Autodesk Inventor part; units mm, degrees
ref_plane "YZ Plane" through (0, 0, 0) normal (1, 0, 0) x (0, 1, 0)
ref_plane "XZ Plane" through (0, 0, 0) normal (0, 1, 0) x (-1, 0, 0)
ref_plane "XY Plane" through (0, 0, 0) normal (0, 0, 1) x (1, 0, 0)
sketch "Sketch1" plane through (0, 0, 0) normal (0, 0, 1) x (1, 0, 0)
  line L0 (0, 0) -> (-1.5, 0)
  line L1 (-1.5, 0) -> (-1.5, 7)
  line L2 (-1.5, 7) -> (-1.5, 7)
  line L3 (-1.5, 7) -> (-1.5, 8)
  line L4 (-1.5, 8) -> (-3, 8)
  line L5 (-3, 8) -> (-3, 10)
  line L6 (-3, 10) -> (0, 10)
  line L7 (0, 10) -> (0, 0)
  dimension "d0" = 2
  dimension "d1" = 3
  dimension "d2" = 1.5
  dimension "d3" = 0
  dimension "d4" = 1
  dimension "d5" = 10
  dimension "d6" = 90
revolve "Revolution1" add sketch "Sketch1" angle 360 about axis through (0, 10, 0) along (0, -1, 0)
thread "Thread1"
sketch "Sketch2" plane through (0, 10, 0) normal (0, 1, 0) x (1, 0, 0)
  line L0 (5, 0.35) -> (-5, 0.35)
  line L1 (-5, 0.35) -> (-5, -0.35)
  line L2 (-5, -0.35) -> (5, -0.35)
  line L3 (5, -0.35) -> (5, 0.35)
  line L4 (5, 0.35) -> (-5, -0.35) construction
  line L5 (-5, 0.35) -> (5, -0.35) construction
  point P0 (0, 0)
  dimension "d10" = 10
  dimension "d11" = 0.7
fillet "Fillet1" radius 0.25 1 edges at (3, 10, 0)
extrude "Extrusion2" cut sketch "Sketch2" against normal blind 0.7
fillet "Fillet2" radius 0.3 1 edges at (1.5, 8, 0)
properties part number "TorsionOscillator-Screw-M3-Brass-CheeseHead-8mm-Std" material "Brass, Soft Yellow"
Part model, mm, in its own coordinate system. A direction names the side the tool comes from. Give positions to 0.01 mm unless a question says otherwise; leave off trailing zeros. Order: outer loops, then holes, each group sorted by start corner. A loop starts at its lowest first (then second) coordinate and runs counter-clockwise, first axis right, second up. Notation, with made-up numbers: (20, 68) - (78, 68) arc R26 cw to (78, 85) - close; hole circle Ø6 at (63.5, -19.75). An arc over 180 degrees is marked (long way). One line per question, with ' | ' between items.
1. Band-saw the part on A-A on x = 0. List the corners of the cut face in (y, z).
Filled in:
outline: (0, -1.5) - (7.7, -1.5) arc R0.3 cw to (8, -1.8) - (8, -3) - (9.75, -3) arc R0.25 ccw to (10, -2.75) - (10, -0.35) - (9.3, -0.35) - (9.3, 0.35) - (10, 0.35) - (10, 2.75) arc R0.25 ccw to (9.75, 3) - (8, 3) - (8, 1.8) arc R0.3 cw to (7.7, 1.5) - (0, 1.5) - close
2. Drill centre lines: probe 1 along Y at (x, z) = (-1.05, 1.75); probe 2 along Y at (x, z) = (-0.9, 0); probe 3 along X at (y, z) = (7.5, 0.75). Where is each one in solid material? Low to high.
Filled in:
probe 1: 8 to 10 | probe 2: 0 to 9.3 | probe 3: -1.3 to 1.3
3. Band-saw the part on C-C on y = 1. List the corners of the cut face in (x, z), then the cut area to 3 significant figures.
Filled in:
outline: circle Ø3 at (0, 0) | area: 7.07 mm²
4. Band-saw the part on B-B on z = 0. List the corners of the cut face in (x, y).
Filled in:
outline: (-3, 8) - (-1.8, 8) arc R0.3 cw to (-1.5, 7.7) - (-1.5, 0) - (1.5, 0) - (1.5, 7.7) arc R0.3 cw to (1.8, 8) - (3, 8) - (3, 9.3) - (-3, 9.3) - close
5. Band-saw the part on D-D on y = 9. List the corners of the cut face in (x, z).
Filled in:
outline: circle Ø6 at (0, 0)
6. Which spindle directions (+Z, -Z, +X, -X, +Y, -Y) get a long thin tool onto all of the face, cutting with end or side? Do faces 1 (the face through (0, 8, 2)), 2 (the face through (-2.77, 8.89, -1.15)). Say none if no direction does.
Filled in:
face 1: -Y | face 2: +Y, -Y
7. Drop flat-ended pins along their axis: P1, Ø3, axis at y = 5.5, z = -1.5, coming from the +X side; P2, Ø3, axis at x = -0.5, y = 1.5, coming from the -Z side; P3, Ø3, axis at x = 1.5, z = 0.5, coming from the -Y side; P4, Ø3, axis at x = -2, y = 2.5, coming from the -Z side. Give the stop position or say it passes through.
Filled in:
P1: x = 1.5 | P2: z = -1.5 | P3: y = 0 | P4: z = -1.41
